Geometry check sheet. Reference: drawing and pictorial views, mm from the part's lowest x, y, z. Give positions to 0.01 mm unless a question says otherwise; leave off trailing zeros. Write each loop counter-clockwise with the first axis right and the second up, starting at its lowest first coordinate (ties: lowest second). Pieces come first, ordered by that corner, then holes.
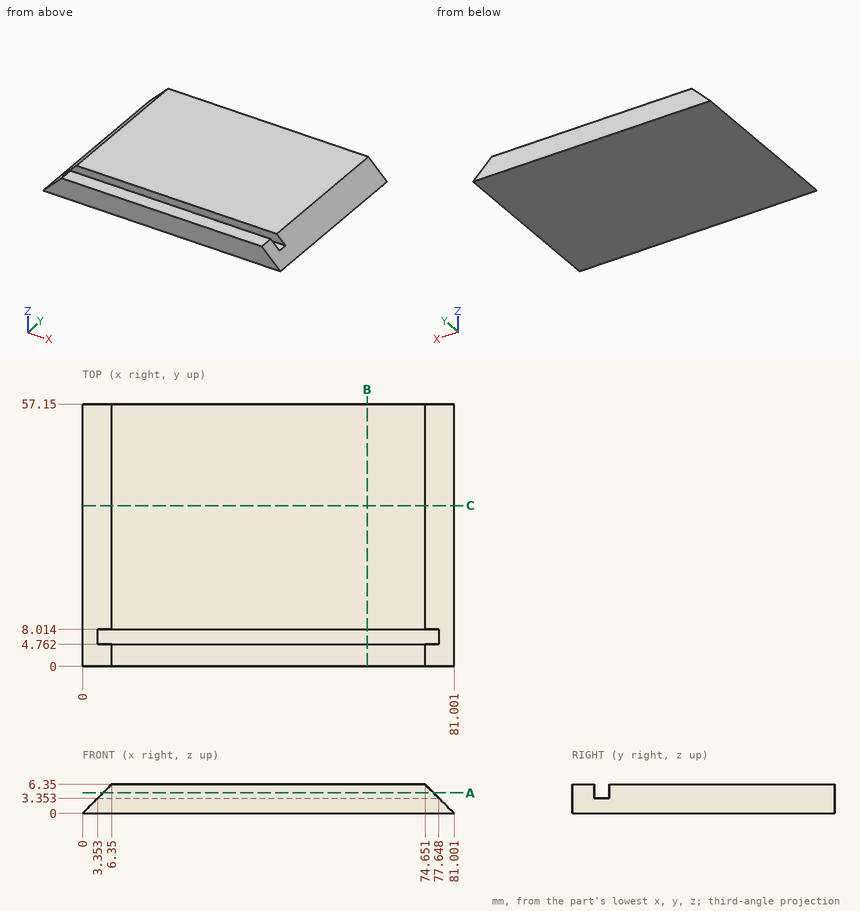
Item 1: Depth check by flat-ended pin: pin 1 (1.6 mm diameter, centred on x = 37, y = 7, fed in from +Z). Enter the tip coordinate at first touch or a pass-through.
Answer key:
pin 1: stops at z = 3.35
Item 2: Scan lines: line 1 along Y through (x, z) = (63, 5.25); line 2 along Z through (x, y) = (12.5, 5); line 3 along X through (y, z) = (8.5, 1.75). Record each from-to range of solid material in increasing order.
Answer key:
line 1: y = 0 to 4.76, 8.01 to 57.15
line 2: z = 0 to 3.35
line 3: x = 1.75 to 79.25
Item 3: Sectioned sample at A-A on z = 4.5. Record the cut outline in (x, y), then the cut area to 3 significant figures.
Answer key:
outline: (4.5, 0) - (76.5, 0) - (76.5, 4.76) - (4.5, 4.76) - close; (4.5, 8.01) - (76.5, 8.01) - (76.5, 57.15) - (4.5, 57.15) - close
area: 3,880 mm2
Item 4: Sectioned sample at C-C on y = 35. Record the cut outline in (x, z), then the cut area to 3 significant figures.
Answer key:
outline: (0, 0) - (81, 0) - (74.65, 6.35) - (6.35, 6.35) - close
area: 474 mm2
Item 5: Sectioned sample at B-B on x = 62. Record the cut outline in (y, z), then the cut area to 3 significant figures.
Answer key:
outline: (0, 0) - (57.15, 0) - (57.15, 6.35) - (8.01, 6.35) - (8.01, 3.35) - (4.76, 3.35) - (4.76, 6.35) - (0, 6.35) - close
area: 353 mm2
